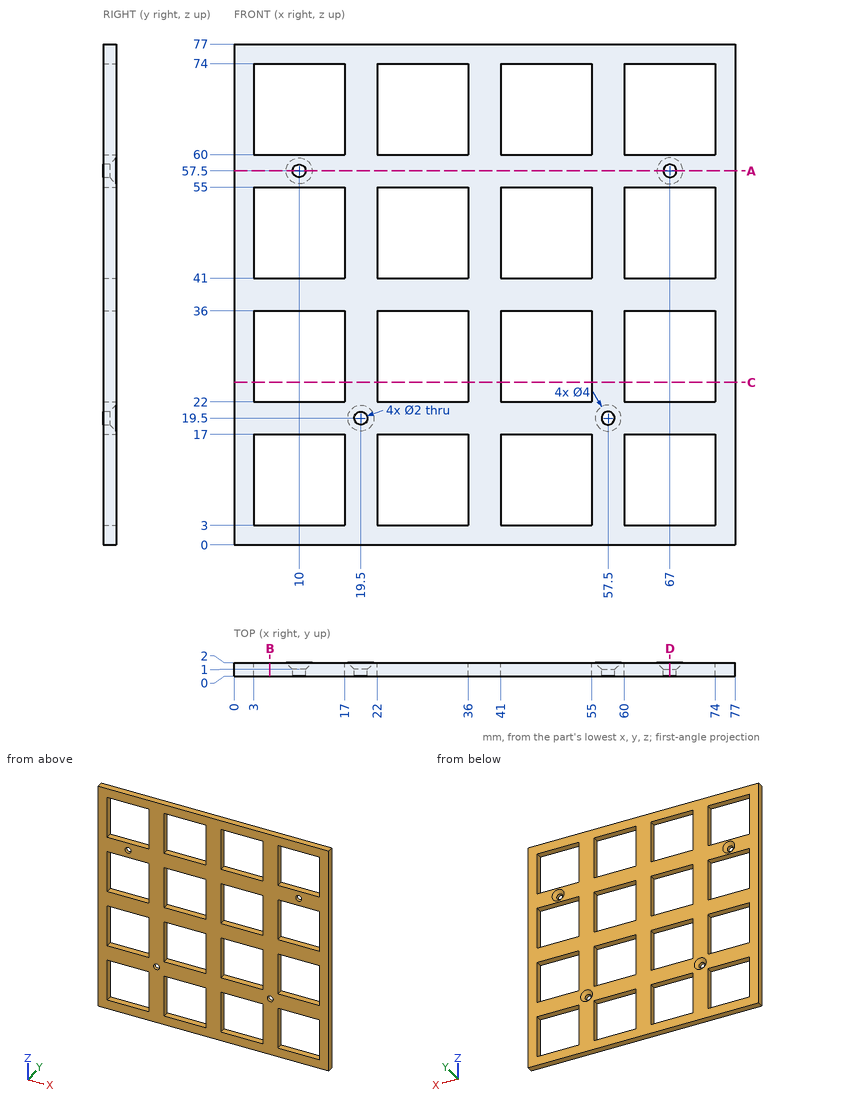
Print and shaded views of the part. All mm, measured from the part's lowest x, y and z. Give positions to 0.01 mm unless a question says otherwise; leave off trailing zeros. Write each loop counter-clockwise with the first axis right and the second up, starting at its lowest first coordinate (ties: lowest second). Pieces come first, ordered by that corner, then holes. Notation, with made-up numbers: (72.25, 49) - (81.25, 49) arc R26 cw to (81.25, 87) - close; hole circle Ø11 at (-22.5, 6). An arc over 180 degrees is marked (long way). Put each result on its own line as item: value.
(1) Saw through at A-A (z = 57.5). List the corners of the cut face in (x, y).
Working result:
outline: (0, 0) - (9, 0) - (9, 1) - (8, 2) - (0, 2) - close; (11, 0) - (66, 0) - (66, 1) - (65, 2) - (12, 2) - (11, 1) - close; (68, 0) - (77, 0) - (77, 2) - (69, 2) - (68, 1) - close
(2) Saw through at D-D (x = 67). List the corners of the cut face in (y, z).
Working result:
outline: (0, 0) - (2, 0) - (2, 3) - (0, 3) - close; (0, 17) - (2, 17) - (2, 22) - (0, 22) - close; (0, 36) - (2, 36) - (2, 41) - (0, 41) - close; (0, 55) - (2, 55) - (2, 55.5) - (1, 56.5) - (0, 56.5) - close; (0, 58.5) - (1, 58.5) - (2, 59.5) - (2, 60) - (0, 60) - close; (0, 74) - (2, 74) - (2, 77) - (0, 77) - close
(3) Saw through at B-B (x = 5.5). List the corners of the cut face in (y, z), then the cut area to 3 significant figures.
Working result:
outline: (0, 0) - (2, 0) - (2, 3) - (0, 3) - close; (0, 17) - (2, 17) - (2, 22) - (0, 22) - close; (0, 36) - (2, 36) - (2, 41) - (0, 41) - close; (0, 55) - (2, 55) - (2, 60) - (0, 60) - close; (0, 74) - (2, 74) - (2, 77) - (0, 77) - close
area: 42.0 mm^2
(4) Drop flat-ended pins along their axis: pin 1 Ø0.6 at (x, y) = (50, 1) entering from -Z; pin 2 Ø3 at (x, z) = (57.5, 19.5) entering from +Y. Give the stop position or say it passes through.
Working result:
pin 1: z = 0
pin 2: y = 1.5
(5) Saw through at C-C (z = 25). List the corners of the cut face in (x, y), then the cut area to 3 significant figures.
Working result:
outline: (0, 0) - (3, 0) - (3, 2) - (0, 2) - close; (17, 0) - (22, 0) - (22, 2) - (17, 2) - close; (36, 0) - (41, 0) - (41, 2) - (36, 2) - close; (55, 0) - (60, 0) - (60, 2) - (55, 2) - close; (74, 0) - (77, 0) - (77, 2) - (74, 2) - close
area: 42.0 mm^2
(6) Wall check: L1, parallel to X at y = 0.25, z = 19.5; L2, parallel to Z at x = 62, y = 0.9. Give the ranges that are in metal, low to high.
Working result:
L1: 0 to 18.5, 20.5 to 56.5, 58.5 to 77
L2: 0 to 3, 17 to 22, 36 to 41, 55 to 60, 74 to 77
